Autodesk Inventor part; units mm, degrees
ref_plane "YZ Plane" through (0, 0, 0) normal (1, 0, 0) x (0, 1, 0)
ref_plane "XZ Plane" through (0, 0, 0) normal (0, 1, 0) x (-1, 0, 0)
ref_plane "XY Plane" through (0, 0, 0) normal (0, 0, 1) x (1, 0, 0)
sketch "Sketch1" plane through (0, 0, 0) normal (0, 1, 0) x (-1, 0, 0)
  line L0 (0, 0) -> (7.366, 0) construction
  line L1 (7.366, 0) -> (3.683, -6.3791)
  line L2 (3.683, -6.3791) -> (-3.683, -6.3791)
  line L3 (-3.683, -6.3791) -> (-7.366, 0)
  line L4 (-7.366, 0) -> (-3.683, 6.3791)
  line L5 (-3.683, 6.3791) -> (3.683, 6.3791)
  line L6 (3.683, 6.3791) -> (7.366, 0)
  dimension "d3" = 7.366
extrude "Extrusion1" add sketch "Sketch1" along normal blind 127
properties part number "hex shaft for wheels"
The model under review builds one solid part; all positions refer to its coordinate system, in mm. Coordinates: 2 decimals unless noted, no trailing zeros. Write each loop counter-clockwise with the first axis right and the second up, starting at its lowest first coordinate (ties: lowest second). Pieces come first, ordered by that corner, then holes. Notation, with made-up numbers: (65, 19.25) - (92, 19.25) arc R15 ccw to (92, 45.25) - close; hole circle Ø1 at (14, -18). An arc over 180 degrees is marked (long way). Answer in a Markdown table with one row per item. Add a question column.
Q1. Consider section A-A on y = 49. Give the boundary of the cut face in (x, z), then the cut area to 3 significant figures.
Q2. Consider section C-C on x = -5. Give the boundary of the cut face in (y, z).
Q3. Draft analysis for pull direction Y (two halves, no side actions). For faces 1 (the face through (0, 127, 0)), 2 (the face through (0, 63, 6.379)), 3 (the face through (0, 0, 0)), state which applies: +Y half, -Y half, draft (parallel to the pull), parting line (faces both ways), or undercut.
Q4. Consider section B-B on z = -2. Give the boundary of the cut face in (x, y).
Q5. To check wall thickness, follow line 1 along X through (y, z) = (48, 3.75); line 2 along Z through (x, y) = (4.25, 23.5); line 3 along X through (y, z) = (57.5, 4.75). State the ranges of each line that lie inside material, in increasing order. Write a range as from..to.
Answers below:
| question | item | result |
|---|---|---|
| 1 | outline | (-7.37, 0) - (-3.68, -6.38) - (3.68, -6.38) - (7.37, 0) - (3.68, 6.38) - (-3.68, 6.38) - close |
| 1 | area | 141 mm² |
| 2 | outline | (0, -4.1) - (127, -4.1) - (127, 4.1) - (0, 4.1) - close |
| 3 | face 1 | +Y half |
| 3 | face 2 | draft |
| 3 | face 3 | -Y half |
| 4 | outline | (-6.21, 0) - (6.21, 0) - (6.21, 127) - (-6.21, 127) - close |
| 5 | line 1 | -5.2..5.2 |
| 5 | line 2 | -5.4..5.4 |
| 5 | line 3 | -4.62..4.62 |
